Autodesk Fusion 360 part; units mm, degrees
sketch "3D-printed conduit top outline" plane through (0, 0, 0) normal (0, 1, 0) x (1, 0, 0)
  line L0 (0, 0) -> (16, 0)
  line L1 (16, 0) -> (16, -2)
  line L2 (16, -2) -> (0, -2)
  line L3 (0, -2) -> (0, 0)
  dimension "d7" = 16
  dimension "d8" = 2
extrude "Extrude1" add sketch "3D-printed conduit top outline" along normal blind 161
sketch "Magnet holes" plane through (0, 0, 2) normal (0, 0, 1) x (-1, 0, 0)
  line L0 (0, 0) -> (-16, 0)
  line L1 (-16, 0) -> (-16, -161)
  line L2 (-16, -161) -> (0, -161)
  line L3 (0, -161) -> (0, 0)
  circle A0 centre (-2.5, -2.5) radius 2.5
  circle A1 centre (-13.5, -2.5) radius 2.5
  circle A2 centre (-2.5, -2.5) radius 1.75
  circle A3 centre (-13.5, -2.5) radius 1.75
  circle A4 centre (-2.5, -54.5) radius 1.75
  circle A5 centre (-2.5, -54.5) radius 2.5
  circle A6 centre (-13.5, -54.5) radius 2.5
  circle A7 centre (-13.5, -54.5) radius 1.75
  circle A8 centre (-2.5, -106.5) radius 1.75
  circle A9 centre (-2.5, -106.5) radius 2.5
  circle A10 centre (-13.5, -106.5) radius 2.5
  circle A11 centre (-13.5, -106.5) radius 1.75
  circle A12 centre (-2.5, -158.5) radius 1.75
  circle A13 centre (-2.5, -158.5) radius 2.5
  circle A14 centre (-13.5, -158.5) radius 2.5
  circle A15 centre (-13.5, -158.5) radius 1.75
  dimension "d11" = 5
  dimension "d12" = 5
  dimension "d13" = 3.5
  dimension "d14" = 3.5
  dimension "d17" = 0
  dimension "d18" = -156
extrude "Extrude2" cut sketch "Magnet holes" against normal blind 1 contours A2 | A3 | A4 | A7 | A8 | A11 | A12 | A15
sketch "Support rib" plane through (0, 0, 2) normal (0, 0, 1) x (-1, 0, 0)
  line L0 (0, 0) -> (-16, 0)
  line L1 (-16, 0) -> (-16, -161)
  line L2 (-16, -161) -> (0, -161)
  line L3 (0, -161) -> (0, 0)
  circle A0 centre (-13.5, -158.5) radius 1.75
  circle A1 centre (-13.5, -54.5) radius 1.75
  circle A2 centre (-2.5, -2.5) radius 1.75
  circle A3 centre (-2.5, -106.5) radius 1.75
  circle A4 centre (-2.5, -158.5) radius 1.75
  circle A5 centre (-2.5, -54.5) radius 1.75
  circle A6 centre (-13.5, -2.5) radius 1.75
  circle A7 centre (-13.5, -106.5) radius 1.75
  line L4 (-5.5, 0) -> (-10.5, 0)
  line L5 (-10.5, 0) -> (-10.5, -161)
  line L6 (-10.5, -161) -> (-5.5, -161)
  line L7 (-5.5, -161) -> (-5.5, 0)
  dimension "d23" = 5
  dimension "d24" = 5.5
  dimension "d25" = 5.5
extrude "Extrude3" add sketch "Support rib" along normal blind 3 contours L0 L2 L4 L5 L6 L7
chamfer "Chamfer1" distance 0.5 angle 45 2 edges at (5.5, 80.5, 5) (10.5, 80.5, 5)
equation "conduit_length = 161 mm"
equation "conduit_width = 16 mm"
equation "conduit_wall_thickness = 2 mm"
equation "magnet_diameter = 3 mm"
equation "magnet_height = 1 mm"
equation "d7 = conduit_width"
equation "d8 = conduit_wall_thickness"
equation "d9 = conduit_length"
equation "d11 = magnet_diameter + 2 mm"
equation "d12 = magnet_diameter + 2 mm"
equation "d13 = magnet_diameter + 0.5 mm"
equation "d14 = magnet_diameter + 0.5 mm"
equation "d18 = -conduit_length + magnet_diameter + 2 mm"
equation "rib_width = 5 mm"
equation "rib_height = 3 mm"
equation "d23 = rib_width"
equation "d24 = ( conduit_width - rib_width ) / 2"
equation "d26 = rib_height"
equation "rib_chamfer = 0.5 mm"
equation "d29 = rib_chamfer"
The model under review builds one solid part; all positions refer to its coordinate system, in mm. A direction names the side the tool comes from. Round coordinates to 2 decimals unless told otherwise and drop trailing zeros. Write each loop counter-clockwise with the first axis right and the second up, starting at its lowest first coordinate (ties: lowest second). Pieces come first, ordered by that corner, then holes. Notation, with made-up numbers: M 67,-22 L 104,-22 A32 cw 104,4 Z; hole C 44.25,64 d8. An arc over 180 degrees is marked long. Use CSV: the item, a comma, the result in double quotes. Start each with the question number.
(1) We need section A-A, the plane y = 54.5. State the section outline as (x, z) points.
(2) Tool access review of faces 1 (the face through (8, 79, 5)), 2 (the face through (14, 158, 1)), 3 (the face through (5.5, 82, 3)): name each direction out of +Z, -Z, +X, -X, +Y, -Y from which nothing blocks a thin tool from reaching the whole face with its end or side.
(3) Clearance check with flat-ended pins moving along their axes: P1, Ø1.6, axis at x = 14.5, y = 49.5, coming from the +Z side; P2, Ø1, axis at x = 12.5, y = 54.5, coming from the +Z side. State where each tip first meets the part, or that it passes through.
(4) We need section B-B, the plane x = 13.5. State the section outline as (y, z) points.
(5) We need section C-C, the plane y = 85.5. State the section outline as (x, z) points, then the cut area to 4 significant figures.
(6) For line 1 along Y through (x, z) = (13.5, 1.4); line 2 along X through (y, z) = (106.5, 1.25); line 3 along X through (y, z) = (29, 3.2), list the stretches that pass through material, from the lowest coordinate up.
(7) The part is to be moulded in two halves that separate along Y. For faces 4 (the face through (8, 161, 2)), 5 (the face through (13, 79, 2)), 6 (the face through (3, 54, 1)), say which applies: +Y half, -Y half, draft (parallel to the pull), parting line (faces both ways), or undercut.
Findings:
1,outline,"M 0,0 L 16,0 L 16,2 L 15.25,2 L 15.25,1 L 11.75,1 L 11.75,2 L 10.5,2 L 10.5,4.5 L 10,5 L 6,5 L 5.5,4.5 L 5.5,2 L 4.25,2 L 4.25,1 L 0.75,1 L 0.75,2 L 0,2 Z"
2,face 1,"+Z, +X, -X, +Y, -Y"
2,face 2,"+Z"
2,face 3,"+Z, -X, +Y, -Y"
3,P1,"z = 2"
3,P2,"z = 1"
4,outline,"M 0,0 L 161,0 L 161,2 L 160.25,2 L 160.25,1 L 156.75,1 L 156.75,2 L 108.25,2 L 108.25,1 L 104.75,1 L 104.75,2 L 56.25,2 L 56.25,1 L 52.75,1 L 52.75,2 L 4.25,2 L 4.25,1 L 0.75,1 L 0.75,2 L 0,2 Z"
5,outline,"M 0,0 L 16,0 L 16,2 L 10.5,2 L 10.5,4.5 L 10,5 L 6,5 L 5.5,4.5 L 5.5,2 L 0,2 Z"
5,area,"46.75 mm^2"
6,line 1,"0 to 0.75, 4.25 to 52.75, 56.25 to 104.75, 108.25 to 156.75, 160.25 to 161"
6,line 2,"0 to 0.75, 4.25 to 11.75, 15.25 to 16"
6,line 3,"5.5 to 10.5"
7,face 4,"+Y half"
7,face 5,"draft"
7,face 6,"undercut"
